```python
from build123d import *

# Parameters (mm, degrees)
F1_DEPTH = 22.5
F2_R     = 2.5
F3_DEPTH = 5.001
F4_R     = 2.5
F5_DEPTH = 5.001
F7_DEPTH = 22.501


with BuildPart() as f1:
    # F0 (on Front) → F1 (new body)
    with BuildSketch(Plane.XZ):
        Polygon((-18.470997, -15.365735), (-18.272383, -20.357819), (41.727616, -20.365735), (41.727616, -15.365735), (29.227616, -15.365735), (29.227616, -2.865735), (-5.970997, -2.865735), (-5.970997, -15.365735), align=None)
    extrude(amount=F1_DEPTH)

    # F2 (on face) → F3 (cut, through all)
    with BuildSketch(Plane.XY.offset(-15.365735)):
        with Locations((35.477616, -11.25)):
            Circle(F2_R)
    extrude(amount=-F3_DEPTH, mode=Mode.SUBTRACT)

    # F4 (on face) → F5 (cut, through all)
    with BuildSketch(Plane.XY.offset(-15.365735)):
        with Locations((-12.220997, -11.25)):
            Circle(F4_R)
    extrude(amount=-F5_DEPTH, mode=Mode.SUBTRACT)

    # F6 (on face) → F7 (cut, through all)
    with BuildSketch(Plane.XZ.offset(22.5)):
        with BuildLine():
            ThreePointArc((0, -2.865735), (3.599998, -10.703488), (11.62831, -13.855716))
            ThreePointArc((11.62831, -13.855716), (20.377936, -11.151829), (24.277631, -2.865735))
            Line((24.277631, -2.865735), (11.62831, -2.865735))
            Line((11.62831, -2.865735), (0, -2.865735))
        make_face()
    extrude(amount=-F7_DEPTH, mode=Mode.SUBTRACT)


solid = f1.part
```
The model under review builds one solid part; all positions refer to its coordinate system, in mm. A direction names the side the tool comes from. Round coordinates to 2 decimals unless told otherwise and drop trailing zeros. Order: outer loops, then holes, each group sorted by start corner. A loop starts at its lowest first (then second) coordinate and runs counter-clockwise, first axis right, second up. Notation, with made-up numbers: (-19, -13) -> (37, -13) arc R21 cw to (37, 20) -> close; hole circle Ø9 at (55.5, 28.25). An arc over 180 degrees is marked (long way). Use a Markdown table: item, result.
Q1. Tool access review of faces 4 (the cylindrical face through (3.51, -11.41, -10.62)), 5 (the flat face through (-12.1, -8.6, -15.366)), 6 (the flat face through (29.228, -11, -9)): name each direction out of +Z, -Z, +X, -X, +Y, -Y from which nothing blocks a thin tool from reaching the whole face with its end or side.
Values:
| item | result |
|---|---|
| face 4 | +Z, +Y, -Y |
| face 5 | +Z, -X, +Y, -Y |
| face 6 | +Z, +X, +Y, -Y |
Q2. Clearance check with flat-ended pins moving along their axes: P1, Ø3, axis at x = -8.5, z = -10.5, coming from the -Y side; P2, Ø1.5, axis at y = -11, z = -18, coming from the -X side; P3, Ø6.5, axis at x = -12.22, y = -11.25, coming from the -Z side; P4, Ø6, axis at y = -12.5, z = -7.5, coming from the +X side. State where each tip first meets the part, or that it passes through.
Values:
| item | result |
|---|---|
| P1 | passes through |
| P2 | stops at x = -18.4 |
| P3 | stops at z = -20.36 |
| P4 | stops at x = 29.23 |
Q3. We need section C-C on x = 36.5. Write out the cut boundary in (y, z).
Values:
| item | result |
|---|---|
| outline | (-22.5, -20.37) -> (-13.53, -20.37) -> (-13.53, -15.37) -> (-22.5, -15.37) -> close; (-8.97, -20.37) -> (0, -20.37) -> (0, -15.37) -> (-8.97, -15.37) -> close |
Q4. We need section B-B on z = -6.75. Write out the cut boundary in (x, y), then the cut area to 3 significant figures.
Values:
| item | result |
|---|---|
| outline | (-5.97, -22.5) -> (0.87, -22.5) -> (0.87, 0) -> (-5.97, 0) -> close; (23.49, -22.5) -> (29.23, -22.5) -> (29.23, 0) -> (23.49, 0) -> close |
| area | 283 mm^2 |
Q5. We need section A-A on y = -11.25. Write out the cut boundary in (x, z).
Values:
| item | result |
|---|---|
| outline | (-18.47, -15.37) -> (-18.27, -20.36) -> (-14.72, -20.36) -> (-14.72, -15.37) -> close; (-9.72, -20.36) -> (32.98, -20.36) -> (32.98, -15.37) -> (29.23, -15.37) -> (29.23, -2.87) -> (24.28, -2.87) arc R11.34 cw to (11.63, -13.86) arc R11.54 cw to (0, -2.87) -> (-5.97, -2.87) -> (-5.97, -15.37) -> (-9.72, -15.37) -> close; (37.98, -20.37) -> (41.73, -20.37) -> (41.73, -15.37) -> (37.98, -15.37) -> close |
Q6. Mouldability with a two-part tool opening along X and no side actions: class faces 1 (the cylindrical face through (20.278, -11.408, -11.238)), 2 (the flat face through (41.728, -11, -18)), 3 (the flat face through (-5.971, -11, -9)) as +X half, -X half, draft (parallel to the pull), parting line (faces both ways), or undercut.
Values:
| item | result |
|---|---|
| face 1 | undercut |
| face 2 | +X half |
| face 3 | -X half |
Q7. We need section D-D on z = -17. Write out the cut boundary in (x, y).
Values:
| item | result |
|---|---|
| outline | (-18.41, -22.5) -> (41.73, -22.5) -> (41.73, 0) -> (-18.41, 0) -> close; hole circle Ø5 at (-12.22, -11.25); hole circle Ø5 at (35.48, -11.25) |
Q8. For line 1 (X direction, y = -11.25, z = -17.4); line 2 (X direction, y = -11.25, z = -18.5); line 3 (Z direction, x = 26, y = -18.5), list the stretches that pass through material, from the lowest coordinate up.
Values:
| item | result |
|---|---|
| line 1 | x = -18.39 to -14.72, -9.72 to 32.98, 37.98 to 41.73 |
| line 2 | x = -18.35 to -14.72, -9.72 to 32.98, 37.98 to 41.73 |
| line 3 | z = -20.36 to -2.87 |
